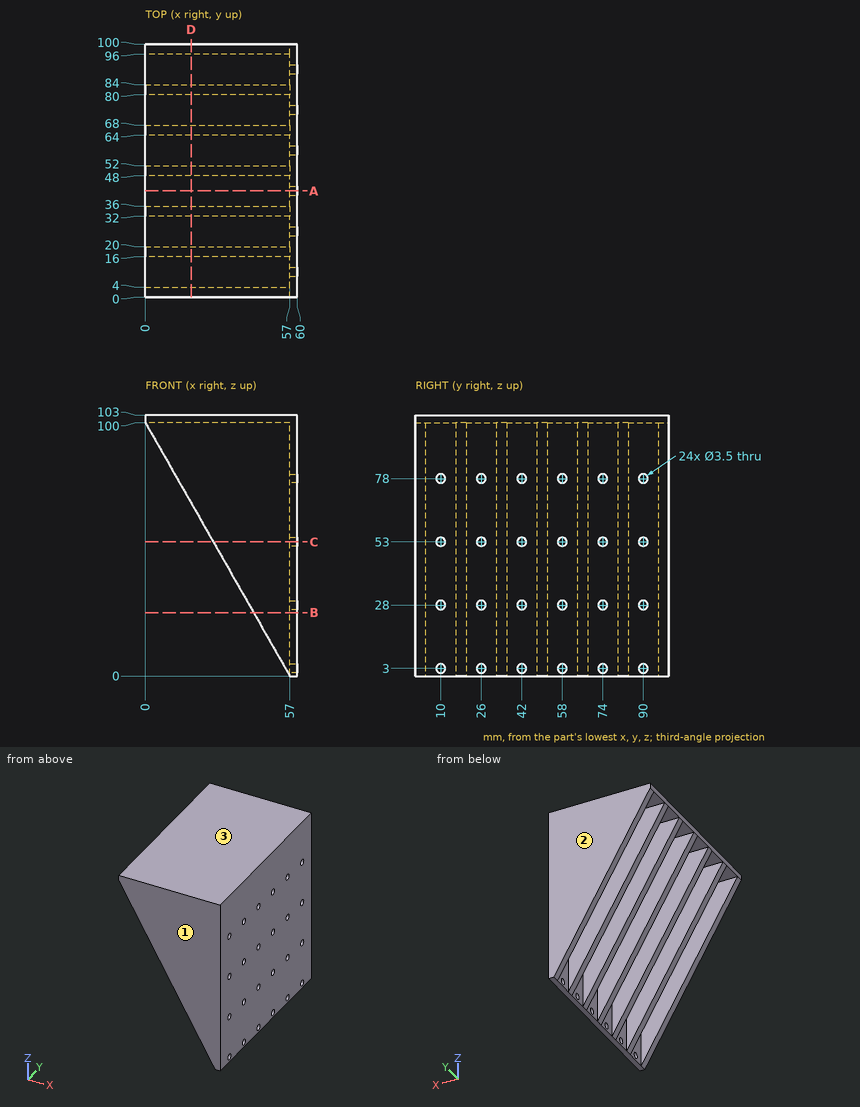
Here's the drawing with two shaded views (mm, measured from the low corner). I have some questions. Give positions to 0.01 mm unless a question says otherwise; leave off trailing zeros. Loops run counter-clockwise (first coordinate to the right, second up) from the corner with the lowest first, then second, coordinate; pieces in that order, holes last. Notation, with made-up numbers: M -28,73.25 L 20,73.25 A17 cw 20,98.25 Z; hole C -10.75,-16 d11. An arc over 180 degrees is marked long. Answer in a Markdown table with one row per item.
1. If I drill on line 1 along X through (y, z) = (53, 7.5); line 2 along Z through (x, y) = (22, 92); line 3 along X through (y, z) = (17.5, 57.5) (3 decimals), over which ranges is the centre line in solid material (lowest first)?
Taken from the geometry:
| item | result |
|---|---|
| line 1 | x = 57 to 60 |
| line 2 | z = 100 to 103 |
| line 3 | x = 24.225 to 60 |
2. Suppose I cut it at D-D on x = 18. Write out the boundary of the cut face in (y, z), plus the area to 3 significant figures.
Taken from the geometry:
| item | result |
|---|---|
| outline | M 0,68.42 L 4,68.42 L 4,100 L 16,100 L 16,68.42 L 20,68.42 L 20,100 L 32,100 L 32,68.42 L 36,68.42 L 36,100 L 48,100 L 48,68.42 L 52,68.42 L 52,100 L 64,100 L 64,68.42 L 68,68.42 L 68,100 L 80,100 L 80,68.42 L 84,68.42 L 84,100 L 96,100 L 96,68.42 L 100,68.42 L 100,103 L 0,103 Z |
| area | 1,180 mm² |
3. Suppose I cut it at C-C on z = 53. Count the separate pieces of the cut face and the enclosed holes in it, plus the area to 3 significant figures.
Taken from the geometry:
| item | result |
|---|---|
| separate pieces | 7 |
| enclosed holes | 0 |
| area | 1,080 mm² |
4. Suppose I cut it at A-A on y = 42. Write out the boundary of the cut face in (x, z), plus the area to 3 significant figures.
Taken from the geometry:
| item | result |
|---|---|
| outline | M 0,100 L 57,100 L 57,79.75 L 60,79.75 L 60,103 L 0,103 Z; M 57,0 L 60,0 L 60,1.25 L 57,1.25 Z; M 57,4.75 L 60,4.75 L 60,26.25 L 57,26.25 Z; M 57,29.75 L 60,29.75 L 60,51.25 L 57,51.25 Z; M 57,54.75 L 60,54.75 L 60,76.25 L 57,76.25 Z |
| area | 438 mm² |
5. Thinking about a two-plate mould opening in Y: for the marked faces 1, 2 and 3, which applies, released by +Y, released by -Y, zero draft, split by the parting line, or undercut?
Taken from the geometry:
| item | result |
|---|---|
| face 1 | released by -Y |
| face 2 | released by +Y |
| face 3 | zero draft |
6. For pin 1 Ø10 at (y, z) = (52.5, 43.5) entering from -X; pin 2 Ø8 at (y, z) = (14.5, 29.5) entering from -X; pin 3 Ø8 at (x, y) = (10, 20.5) entering from -Z; pin 4 Ø3 at (y, z) = (10, 28) entering from -X, each with a flat end and sliding along its axis, tell me the tip position at first contact or that it passes through.
Taken from the geometry:
| item | result |
|---|---|
| pin 1 | stops at x = 29.37 |
| pin 2 | stops at x = 38.07 |
| pin 3 | stops at z = 75.49 |
| pin 4 | passes through |
7. Suppose I cut it at B-B on z = 25. Write out the boundary of the cut face in (x, y), plus the area to 3 significant figures.
Taken from the geometry:
| item | result |
|---|---|
| outline | M 42.75,0 L 60,0 L 60,100 L 42.75,100 L 42.75,96 L 57,96 L 57,84 L 42.75,84 L 42.75,80 L 57,80 L 57,68 L 42.75,68 L 42.75,64 L 57,64 L 57,52 L 42.75,52 L 42.75,48 L 57,48 L 57,36 L 42.75,36 L 42.75,32 L 57,32 L 57,20 L 42.75,20 L 42.75,16 L 57,16 L 57,4 L 42.75,4 Z |
| area | 699 mm² |
